```python
from build123d import *

# Parameters (mm, degrees)
SKETCH1_W           = 40
SKETCH1_H           = 40
SKETCH1_W_2         = 36
SKETCH1_H_2         = 36
BOSS_EXTRUDE1_DEPTH = 80
CUT_EXTRUDE1_REACH  = 93.652
SKETCH2_R           = 4
CUT_EXTRUDE2_REACH  = 93.652
SKETCH3_R           = 4


with BuildPart() as part:
    # Sketch1 → Boss-Extrude1 (new body)
    with BuildSketch(Plane.XY):
        Rectangle(SKETCH1_W, SKETCH1_H)
        Rectangle(SKETCH1_W_2, SKETCH1_H_2, mode=Mode.SUBTRACT)
    extrude(amount=BOSS_EXTRUDE1_DEPTH)

    # Sketch2 → Cut-Extrude1 (cut, up to next)
    with BuildSketch(Plane(origin=(0, 20, 0), x_dir=(1, 0, 0), z_dir=(0, 1, 0)), mode=Mode.PRIVATE) as cut_extrude1_sk1:
        with Locations(Location((0, -20, 0), (0, 0, 270))):
            Circle(SKETCH2_R)
    cut_extrude1_tool1 = extrude(cut_extrude1_sk1.sketch, amount=-CUT_EXTRUDE1_REACH, mode=Mode.PRIVATE) & part.part
    # Sketch2 → Cut-Extrude1 (cut, up to next)
    with BuildSketch(Plane(origin=(0, 20, 0), x_dir=(1, 0, 0), z_dir=(0, 1, 0)), mode=Mode.PRIVATE) as cut_extrude1_sk2:
        with Locations(Location((0, -40, 0), (0, 0, 270))):
            Circle(SKETCH2_R)
    cut_extrude1_tool2 = extrude(cut_extrude1_sk2.sketch, amount=-CUT_EXTRUDE1_REACH, mode=Mode.PRIVATE) & part.part
    add(cut_extrude1_tool1.solids().sort_by_distance((0, 20, 20))[0], mode=Mode.SUBTRACT)
    add(cut_extrude1_tool2.solids().sort_by_distance((0, 20, 40))[0], mode=Mode.SUBTRACT)

    # Sketch3 → Cut-Extrude2 (cut, up to next)
    with BuildSketch(Plane.XZ.offset(20), mode=Mode.PRIVATE) as cut_extrude2_sk1:
        with Locations(Location((0, 20, 0), (0, 0, 90))):
            Circle(SKETCH3_R)
    cut_extrude2_tool1 = extrude(cut_extrude2_sk1.sketch, amount=-CUT_EXTRUDE2_REACH, mode=Mode.PRIVATE) & part.part
    add(cut_extrude2_tool1.solids().sort_by_distance((0, -20, 20))[0], mode=Mode.SUBTRACT)


solid = part.part
```
Build history of the part. All positions in model axes, mm. A direction names the side the tool comes from. Give positions to 0.01 mm unless a question says otherwise; leave off trailing zeros. Loops run counter-clockwise (first coordinate to the right, second up) from the corner with the lowest first, then second, coordinate; pieces in that order, holes last. Notation, with made-up numbers: (-39, 55.25) -> (-4, 55.25) arc R10 cw to (-4, 59.25) -> close; hole circle Ø11 at (43.25, 74). An arc over 180 degrees is marked (long way). One line per question, with ' | ' between items. Start each with the question number.
1) Pin check, flat tips, straight feed: pin 1 (1.5 mm diameter, centred on x = 2, z = 42, fed in from +Y); pin 2 (13 mm diameter, centred on x = 0, z = 20, fed in from +Y); pin 3 (7 mm diameter, centred on x = 0, z = 20, fed in from +Y). Stop position of each tip, or through.
2) Cut at B-B (y = -2). Give the cut face in (x, z).
3) Cut at A-A (x = 0). Give the cut face in (y, z), plus the area to 3 significant figures.
4) Two-plate mould, pull along X, no slides. Class faces 1 (the cylindrical face through (-2.4, 19, 16.8)), 2 (the flat face through (20, 0, 39)), 3 (the flat face through (-2, -19, 80)), 4 (the flat face through (-20, 0, 39)): released by +X, released by -X, zero draft, split by the parting line, or undercut.
5) Cut at C-C (z = 20). Give the cut face in (x, y).
6) Probe L1, parallel to X at y = -3.5, z = 66.5; L2, parallel to X at y = 18.4, z = 40. List the from-to ranges inside material, lowest first.
7) 3-axis set-ups, long thin cutter, end or side, ignore diameter. For faces 5 (the cylindrical face through (2.4, -19, 16.8)), 6 (the cylindrical face through (-2.4, 19, 36.8)), 7 (the flat face through (18, 0, 39)): which of +Z, -Z, +X, -X, +Y, -Y reach the whole face in a straight line?
Return value:
1) pin 1: y = -18 | pin 2: y = 20 | pin 3: through
2) outline: (-20, 0) -> (-18, 0) -> (-18, 80) -> (-20, 80) -> close; (18, 0) -> (20, 0) -> (20, 80) -> (18, 80) -> close
3) outline: (-20, 0) -> (-18, 0) -> (-18, 16) -> (-20, 16) -> close; (-20, 24) -> (-18, 24) -> (-18, 80) -> (-20, 80) -> close; (18, 0) -> (20, 0) -> (20, 16) -> (18, 16) -> close; (18, 24) -> (20, 24) -> (20, 36) -> (18, 36) -> close; (18, 44) -> (20, 44) -> (20, 80) -> (18, 80) -> close | area: 272 mm^2
4) face 1: undercut | face 2: released by +X | face 3: zero draft | face 4: released by -X
5) outline: (-20, -20) -> (-4, -20) -> (-4, -18) -> (-18, -18) -> (-18, 18) -> (-4, 18) -> (-4, 20) -> (-20, 20) -> close; (4, -20) -> (20, -20) -> (20, 20) -> (4, 20) -> (4, 18) -> (18, 18) -> (18, -18) -> (4, -18) -> close
6) L1: -20 to -18, 18 to 20 | L2: -20 to -4, 4 to 20
7) face 5: +Y, -Y | face 6: +Y | face 7: +Z, -Z
